Design review of the part built by this model. Coordinates are the model's own, in mm. Face numbers are marked on the shaded views. A direction names the side the tool comes from. Give positions to 0.01 mm unless a question says otherwise; leave off trailing zeros. Write each loop counter-clockwise with the first axis right and the second up, starting at its lowest first coordinate (ties: lowest second). Pieces come first, ordered by that corner, then holes. Notation, with made-up numbers: (-25.5, 67) -> (-13.5, 67) arc R13 cw to (-13.5, 83) -> close; hole circle Ø5 at (-12.75, 8). An arc over 180 degrees is marked (long way). Use CSV: the item, a comma, the result in double quotes.
```python
from build123d import *

# Parameters (mm, degrees)
FILLET1_R          = 1
SKETCH2_R          = 2
CUT_EXTRUDE1_DEPTH = 10


with BuildPart() as part:
    # Sketch1 → Revolve1 (revolve)
    with BuildSketch(Plane.XY, mode=Mode.PRIVATE) as revolve1_sk:
        Polygon((0, 0), (0, 20), (6, 20), (6, 8), (14, 8), (14, 0), align=None)
    revolve(revolve1_sk.sketch.rotate(Axis((-4, 0, 0), (0, 1, 0)), 90), axis=Axis((-4, 0, 0), (0, 1, 0)))

    # Fillet1
    fillet1_edges = [part.edges().sort_by_distance(p)[0] for p in [
        (-4, 0, 18),
        (-4, 8, 18),
        (-4, 20, 10),
    ]]
    fillet(fillet1_edges, radius=FILLET1_R)

    # Sketch2 → Cut-Extrude1 (cut)
    with BuildSketch(Plane(origin=(0, 0, 0), x_dir=(-1, 0, 0), z_dir=(0, -1, 0))):
        with Locations(Location((18, 0, 0), (0, 0, 90))):
            Circle(SKETCH2_R)
        with Locations(Location((11, -12.124355653, 0), (0, 0, 90))):
            Circle(SKETCH2_R)
        with Locations(Location((-3, -12.124355653, 0), (0, 0, 90))):
            Circle(SKETCH2_R)
        with Locations(Location((-10, 0, 0), (0, 0, 90))):
            Circle(SKETCH2_R)
        with Locations(Location((-3, 12.124355653, 0), (0, 0, 90))):
            Circle(SKETCH2_R)
        with Locations(Location((11, 12.124355653, 0), (0, 0, 90))):
            Circle(SKETCH2_R)
    extrude(amount=-CUT_EXTRUDE1_DEPTH, mode=Mode.SUBTRACT)


solid = part.part
```
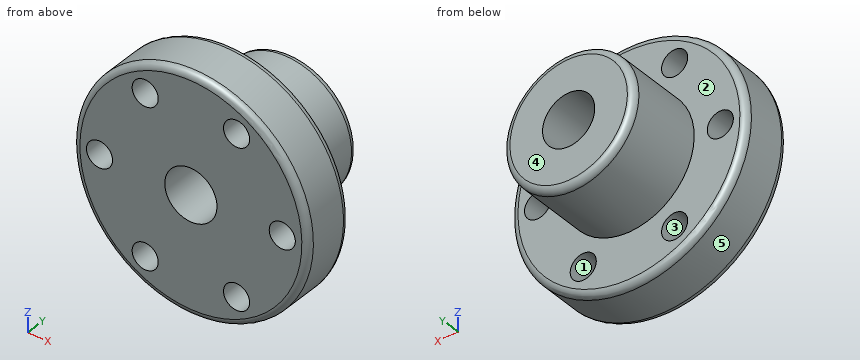
(1) For line 1 along X through (y, z) = (6.75, 0); line 2 along Z through (x, y) = (-11.5, 6.5); line 3 along Z through (x, y) = (-17, 6.5), list the stretches that pass through material, from the lowest coordinate up. Write a range as [from, to].
Established:
line 1,"x = [-22, -20], [-16, -8], [0, 8], [12, 14]"
line 2,"z = [-16.36, -14.06], [-10.19, 10.19], [14.06, 16.36]"
line 3,"z = [-12.45, -1.73], [1.73, 12.45]"
(2) Take a section at A-A (x = -4). Write out the cut boundary in (y, z), then the cut area to 3 significant figures.
Established:
outline,"(0, -17) arc R1 ccw to (1, -18) -> (7, -18) arc R1 ccw to (8, -17) -> (8, -10) -> (19, -10) arc R1 ccw to (20, -9) -> (20, -4) -> (0, -4) -> close; (0, 4) -> (20, 4) -> (20, 9) arc R1 ccw to (19, 10) -> (8, 10) -> (8, 17) arc R1 ccw to (7, 18) -> (1, 18) arc R1 ccw to (0, 17) -> close"
area,"367 mm2"
(3) Take a section at D-D (y = 16.5). Write out the cut boundary in (x, z).
Established:
outline,"circle Ø20 at (-4, 0); hole circle Ø8 at (-4, 0)"
(4) Take a section at B-B (z = 0). Write out the cut boundary in (x, y), then the cut area to 3 significant figures.
Established:
outline,"(-22, 1) arc R1 ccw to (-21, 0) -> (-20, 0) -> (-20, 8) -> (-21, 8) arc R1 ccw to (-22, 7) -> close; (-16, 0) -> (-8, 0) -> (-8, 20) -> (-13, 20) arc R1 ccw to (-14, 19) -> (-14, 8) -> (-16, 8) -> close; (0, 0) -> (8, 0) -> (8, 8) -> (6, 8) -> (6, 19) arc R1 ccw to (5, 20) -> (0, 20) -> close; (12, 0) -> (13, 0) arc R1 ccw to (14, 1) -> (14, 7) arc R1 ccw to (13, 8) -> (12, 8) -> close"
area,"303 mm2"
(5) Tool access review of the marked faces 1 and 2: name each direction out of +Z, -Z, +X, -X, +Y, -Y from which nothing blocks a thin tool from reaching the whole face with its end or side.
Established:
face 1,"+Y, -Y"
face 2,"+Y"
(6) Clearance check with flat-ended pins moving along their axes: pin 1 (8 mm diameter, centred on y = 15, z = 2.5, fed in from +X); pin 2 (5 mm diameter, centred on x = -11, z = -12.12, fed in from +Y); pin 3 (3 mm diameter, centred on x = -1.5, y = 8, fed in from +Z). State where each tip first meets the part, or that it passes through.
Established:
pin 1,"stops at x = 6"
pin 2,"stops at y = 8"
pin 3,"stops at z = 17.95"
(7) Mouldability with a two-part tool opening along X and no side actions: class the marked faces 3, 4 and 5 as +X half, -X half, draft (parallel to the pull), parting line (faces both ways), or undercut.
Established:
face 3,"undercut"
face 4,"draft"
face 5,"parting line"
(8) Take a section at C-C (y = 6.25). Write out the cut boundary in (x, z), then the cut area to 3 significant figures.
Established:
outline,"circle Ø36 at (-4, 0); hole circle Ø4 at (-18, 0); hole circle Ø4 at (-11, -12.12); hole circle Ø4 at (-11, 12.12); hole circle Ø8 at (-4, 0); hole circle Ø4 at (3, -12.12); hole circle Ø4 at (3, 12.12); hole circle Ø4 at (10, 0)"
area,"892 mm2"
